Verification items for the finished model (mm, model axes). A direction names the side the tool comes from. Coordinates: 2 decimals unless noted, no trailing zeros. Loops run counter-clockwise (first coordinate to the right, second up) from the corner with the lowest first, then second, coordinate; pieces in that order, holes last. Notation, with made-up numbers: (63.5, 12) -> (118.5, 12) arc R30 cw to (118.5, 38) -> close; hole circle Ø8 at (7.25, -34). An arc over 180 degrees is marked (long way). Use CSV: the item, a comma, the result in double quotes. Start each with the question number.
```python
from build123d import *

# Parameters (mm, degrees)
SKETCH1_R           = 2.54
SKETCH1_R_2         = 14.2875
BOSS_EXTRUDE1_DEPTH = 3.175


with BuildPart() as part:
    # Sketch1 → Boss-Extrude1 (new body)
    with BuildSketch(Plane.XY):
        with BuildLine():
            Line((0, 0), (0, 50.8))
            Line((0, 50.8), (72.591943157, 50.8))
            Line((72.591943157, 50.8), (97.991943157, 8.381133577))
            ThreePointArc((97.991943157, 8.381133577), (95.945608162, -20.644868853), (67.98549449, -28.702681675))
            Line((67.98549449, -28.702681675), (50.8, -22.829153204))
            Line((50.8, -22.829153204), (50.8, 0))
            Line((50.8, 0), (0, 0))
        make_face()
        with Locations((12.7, 34.42794066)):
            Circle(SKETCH1_R, mode=Mode.SUBTRACT)
        with Locations((25.4, 34.42794066)):
            Circle(SKETCH1_R, mode=Mode.SUBTRACT)
        with Locations((38.1, 34.42794066)):
            Circle(SKETCH1_R, mode=Mode.SUBTRACT)
        with Locations((25.4, 21.72794066)):
            Circle(SKETCH1_R, mode=Mode.SUBTRACT)
        with Locations((38.1, 21.72794066)):
            Circle(SKETCH1_R, mode=Mode.SUBTRACT)
        with Locations((25.4, 9.02794066)):
            Circle(SKETCH1_R, mode=Mode.SUBTRACT)
        with Locations((38.1, 9.02794066)):
            Circle(SKETCH1_R, mode=Mode.SUBTRACT)
        with Locations((12.7, 21.72794066)):
            Circle(SKETCH1_R, mode=Mode.SUBTRACT)
        with Locations((12.7, 9.02794066)):
            Circle(SKETCH1_R, mode=Mode.SUBTRACT)
        with Locations((76.2, -4.667667649)):
            Circle(SKETCH1_R_2, mode=Mode.SUBTRACT)
    extrude(amount=BOSS_EXTRUDE1_DEPTH)


solid = part.part
```
1. Cross-section at D-D, the plane x = 76.2. Record the boundary of the cut face in (y, z) (3 decimals).
2. Release check for a two-part mould opening along X. For faces 1 (the flat face through (85.114, 29.887, 1.565)), 2 (the cylindrical face through (10.828, 23.445, 1.565)), 3 (the flat face through (52, 20, 0)), 4 (the cylindrical face through (35.562, 21.84, 1.565)) record: released by +X, released by -X, zero draft, split by the parting line, or undercut.
3. Scan lines: line 1 (Y direction, x = 25.4, z = 1.25); line 2 (X direction, y = 10, z = 2.7); line 3 (X direction, y = 35, z = 3.05). Record each from-to range of solid material in increasing order.
4. Cross-section at B-B, the plane y = -2. Record the boundary of the cut face in (x, z) (3 decimals), plus the area to 3 significant figures.
5. Cross-section at A-A, the plane x = 38.1. Record the boundary of the cut face in (y, z) (3 decimals), plus the area to 3 significant figures.
6. Depth check by flat-ended pin: pin 1 (10 mm diameter, centred on x = 90, y = -9.5, fed in from -Z); pin 2 (1.6 mm diameter, centred on y = -16, z = 1.5, fed in from -X). Enter the tip coordinate at first touch or a pass-through.
7. Cross-section at C-C, the plane z = 0.65. State how many separate pieces and enclosed holes the cut face has, plus the area to 3 significant figures.
8. Set-up check for faces 5 (the flat face through (50.8, -12, 2)), 6 (the flat face through (36, 50.8, 2)): record each of +Z, -Z, +X, -X, +Y, -Y from which the full face is reachable in a straight line by a thin tool's end or side.
Solution:
1,outline,"(-30.068, 0) -> (-18.955, 0) -> (-18.955, 3.175) -> (-30.068, 3.175) -> close; (9.62, 0) -> (44.774, 0) -> (44.774, 3.175) -> (9.62, 3.175) -> close"
2,face 1,"released by +X"
2,face 2,"undercut"
2,face 3,"zero draft"
2,face 4,"undercut"
3,line 1,"y = 0 to 6.49, 11.57 to 19.19, 24.27 to 31.89, 36.97 to 50.8"
3,line 2,"x = 0 to 10.35, 15.05 to 23.05, 27.75 to 35.75, 40.45 to 97.02"
3,line 3,"x = 0 to 10.23, 15.17 to 22.93, 27.87 to 35.63, 40.57 to 82.05"
4,outline,"(50.8, 0) -> (62.164, 0) -> (62.164, 3.175) -> (50.8, 3.175) -> close; (90.236, 0) -> (101.46, 0) -> (101.46, 3.175) -> (90.236, 3.175) -> close"
4,area,"71.7 mm2"
5,outline,"(0, 0) -> (6.488, 0) -> (6.488, 3.175) -> (0, 3.175) -> close; (11.568, 0) -> (19.188, 0) -> (19.188, 3.175) -> (11.568, 3.175) -> close; (24.268, 0) -> (31.888, 0) -> (31.888, 3.175) -> (24.268, 3.175) -> close; (36.968, 0) -> (50.8, 0) -> (50.8, 3.175) -> (36.968, 3.175) -> close"
5,area,"113 mm2"
6,pin 1,"stops at z = 0"
6,pin 2,"stops at x = 50.8"
7,separate pieces,"1"
7,enclosed holes,"10"
7,area,"4,940 mm2"
8,face 5,"+Z, -Z, -X, -Y"
8,face 6,"+Z, -Z, +X, -X, +Y"
